```python
from build123d import *

# Parameters (mm, degrees)
F0_R      = 3.5
F2_DEPTH  = 9.5
F1_R      = 5
F3_DEPTH  = 15
F4_R      = 50.5
F5_DEPTH  = 70.5
F6_R      = 51.5
F7_DEPTH  = 6.3
F8_R      = 44
F9_DEPTH  = 9.4
F10_R     = 18
F11_DEPTH = 12.1
F15_SIZE  = 5


with BuildPart() as f2:
    # F0 (on Front) → F2 (new body)
    with BuildSketch(Plane.XZ):
        with BuildLine():
            ThreePointArc((-14.031232, 48.771785), (-13.742652, 48.846608), (-13.457391, 48.933231))
            ThreePointArc((-13.457391, 48.933231), (-13.744549, 48.853351), (-14.031232, 48.771785))
        make_face()
        with BuildLine():
            ThreePointArc((-8.47634, 56.366228), (-9.68343, 51.789665), (-13.457391, 48.933231))
            ThreePointArc((-13.457391, 48.933231), (-13.742652, 48.846608), (-14.031232, 48.771785))
            ThreePointArc((-14.031232, 48.771785), (-43.950789, 25.375), (-49.253221, -12.234489))
            ThreePointArc((-49.253221, -12.234489), (-49.173729, -12.521818), (-49.106117, -12.812173))
            ThreePointArc((-49.106117, -12.812173), (-49.69288, -17.508736), (-53.052755, -20.842389))
            ThreePointArc((-53.052755, -20.842389), (-56.724664, -32.75), (-44.576416, -35.523839))
            ThreePointArc((-44.576416, -35.523839), (-40.009451, -34.280929), (-35.648726, -36.121058))
            ThreePointArc((-35.648726, -36.121058), (-35.431077, -36.324789), (-35.221989, -36.537296))
            ThreePointArc((-35.221989, -36.537296), (0, -50.75), (35.221989, -36.537296))
            ThreePointArc((35.221989, -36.537296), (35.431077, -36.324789), (35.648726, -36.121058))
            ThreePointArc((35.648726, -36.121058), (40.009451, -34.280929), (44.576416, -35.523839))
            ThreePointArc((44.576416, -35.523839), (56.724664, -32.75), (53.052755, -20.842389))
            ThreePointArc((53.052755, -20.842389), (49.69288, -17.508736), (49.106117, -12.812173))
            ThreePointArc((49.106117, -12.812173), (49.173729, -12.521818), (49.253221, -12.234489))
            ThreePointArc((49.253221, -12.234489), (43.950789, 25.375), (14.031232, 48.771785))
            ThreePointArc((14.031232, 48.771785), (13.742652, 48.846608), (13.457391, 48.933231))
            ThreePointArc((13.457391, 48.933231), (9.68343, 51.789665), (8.47634, 56.366228))
            ThreePointArc((8.47634, 56.366228), (0, 65.5), (-8.47634, 56.366228))
        make_face()
        with Locations((-49.363448, -28.5)):
            Circle(F0_R, mode=Mode.SUBTRACT)
        with Locations((49.363448, -28.5)):
            Circle(F0_R, mode=Mode.SUBTRACT)
        with Locations((0, 57)):
            Circle(F0_R, mode=Mode.SUBTRACT)
        with BuildLine():
            ThreePointArc((-49.106117, -12.812173), (-49.173729, -12.521818), (-49.253221, -12.234489))
            ThreePointArc((-49.253221, -12.234489), (-49.180517, -12.523547), (-49.106117, -12.812173))
        make_face()
        with BuildLine():
            ThreePointArc((14.031232, 48.771785), (13.744549, 48.853351), (13.457391, 48.933231))
            ThreePointArc((13.457391, 48.933231), (13.742652, 48.846608), (14.031232, 48.771785))
        make_face()
        with BuildLine():
            ThreePointArc((49.106117, -12.812173), (49.180517, -12.523547), (49.253221, -12.234489))
            ThreePointArc((49.253221, -12.234489), (49.173729, -12.521818), (49.106117, -12.812173))
        make_face()
        with BuildLine():
            ThreePointArc((-35.221989, -36.537296), (-35.431077, -36.324789), (-35.648726, -36.121058))
            ThreePointArc((-35.648726, -36.121058), (-35.435968, -36.329804), (-35.221989, -36.537296))
        make_face()
        with BuildLine():
            ThreePointArc((35.648726, -36.121058), (35.431077, -36.324789), (35.221989, -36.537296))
            ThreePointArc((35.221989, -36.537296), (35.435968, -36.329804), (35.648726, -36.121058))
        make_face()
    extrude(amount=-F2_DEPTH)

    # F1 (on face) → F3 (join)
    with BuildSketch(Plane.XZ):
        Circle(F1_R)
    extrude(amount=F3_DEPTH)

    # F4 (on face) → F5 (join)
    with BuildSketch(Plane(origin=(0, 9.5, 0), x_dir=(-1, 0, 0), z_dir=(0, 1, 0))):
        Circle(F4_R)
    extrude(amount=F5_DEPTH)

    # F6 (on face) → F7 (join)
    with BuildSketch(Plane(origin=(0, 80, 0), x_dir=(-1, 0, 0), z_dir=(0, 1, 0))):
        Circle(F6_R)
    extrude(amount=F7_DEPTH)

    # F8 (on face) → F9 (join)
    with BuildSketch(Plane(origin=(0, 86.3, 0), x_dir=(-1, 0, 0), z_dir=(0, 1, 0))):
        Circle(F8_R)
    extrude(amount=F9_DEPTH)

    # F10 (on face) → F11 (join)
    with BuildSketch(Plane(origin=(0, 95.7, 0), x_dir=(-1, 0, 0), z_dir=(0, 1, 0))):
        Circle(F10_R)
    extrude(amount=F11_DEPTH)

    # F15
    f15_edges = [f2.edges().sort_by_distance(p)[0] for p in [
        (44, 95.7, 0),
    ]]
    chamfer(f15_edges, length=F15_SIZE)


solid = f2.part
```
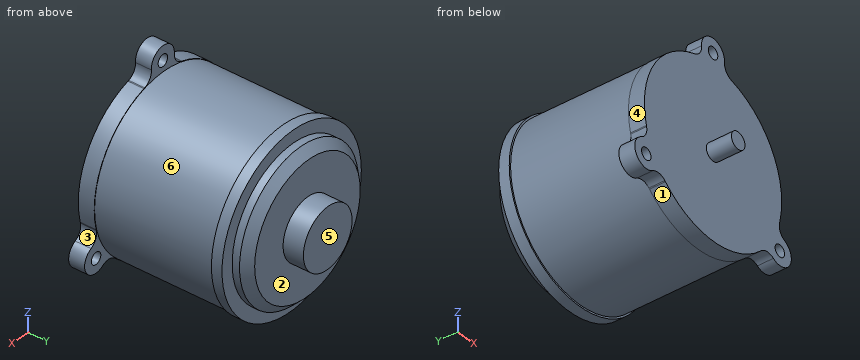
Model file for the job. Use its own axes, mm. Face numbers are marked on the shaded views. A direction names the side the tool comes from. Coordinates: 2 decimals unless noted, no trailing zeros. Loops run counter-clockwise (first coordinate to the right, second up) from the corner with the lowest first, then second, coordinate; pieces in that order, holes last. Notation, with made-up numbers: (53.25, 34.25) - (112.25, 34.25) arc R33 ccw to (112.25, 71.25) - close; hole circle Ø7 at (8, 44.5). An arc over 180 degrees is marked (long way). Write item = value, one per line. Start each with the question number.
Item 1: Wall check: probe 1 along Y at (x, z) = (-10, 34.5); probe 2 along Y at (x, z) = (47.5, -12); probe 3 along Z at (x, y) = (12.5, 52). Give the ranges that are in metal, low to high. Write a range as [from, to].
Item 2: Drop flat-ended pins along their axis: pin 1 Ø1.5 at (x, z) = (-3, -23.5) entering from -Y; pin 2 Ø1.5 at (x, z) = (-12, 36) entering from +Y; pin 3 Ø6 at (x, y) = (38, 22) entering from +Z. Give the stop position or say it passes through.
Item 3: 3-axis set-ups, long thin cutter, end or side, ignore diameter. For the marked faces 1, 2 and 3: which of +Z, -Z, +X, -X, +Y, -Y reach the whole face in a straight line?
Item 4: Saw through at C-C, the plane y = -5.5. List the corners of the cut face in (x, z), then the cut area to 3 significant figures.
Item 5: Pull direction Y, two halves, no side cores. Call the marked faces 4, 5 and 6: +Y half, -Y half, draft (parallel to the pull), parting line (faces both ways), or undercut.
Item 6: Saw through at D-D, the plane z = -28.5. State how many separate pieces and enclosed holes the cut face has, then the cut area to 3 significant figures.
Item 7: Saw through at B-B, the plane z = 0. List the corners of the cut face in (x, y), then the cut area to 3 significant figures.
Answers:
q1.probe_1 = [0, 95.7]
q1.probe_2 = [0, 86.3]
q1.probe_3 = [-48.93, 48.93]
q2.pin_1 = 0
q2.pin_2 = 95.7
q2.pin_3 = 36.4
q3.face_1 = -Z, -Y
q3.face_2 = +Y
q3.face_3 = +X, -Y
q4.outline = circle Ø10 at (0, 0)
q4.area = 78.5 mm2
q5.face_4 = draft
q5.face_5 = +Y half
q5.face_6 = undercut
q6.separate_pieces = 3
q6.enclosed_holes = 0
q6.area = 7,980 mm2
q7.outline = (-51.5, 80) - (-50.5, 80) - (-50.5, 9.5) - (-50.75, 9.5) - (-50.75, 0) - (-5, 0) - (-5, -15) - (5, -15) - (5, 0) - (50.75, 0) - (50.75, 9.5) - (50.5, 9.5) - (50.5, 80) - (51.5, 80) - (51.5, 86.3) - (44, 86.3) - (44, 90.7) - (39, 95.7) - (18, 95.7) - (18, 107.8) - (-18, 107.8) - (-18, 95.7) - (-39, 95.7) - (-44, 90.7) - (-44, 86.3) - (-51.5, 86.3) - close
q7.area = 10,100 mm2
